Autodesk Inventor part; units mm, degrees
ref_plane "YZ Plane" through (0, 0, 0) normal (1, 0, 0) x (0, 1, 0)
ref_plane "XZ Plane" through (0, 0, 0) normal (0, 1, 0) x (-1, 0, 0)
ref_plane "XY Plane" through (0, 0, 0) normal (0, 0, 1) x (1, 0, 0)
sketch "Sketch1" plane through (0, 0, 0) normal (0, 1, 0) x (-1, 0, 0)
  line L0 (10.25, 29) -> (-10.25, 29)
  line L1 (-10.25, 29) -> (-10.25, -29)
  line L2 (-10.25, -29) -> (10.25, -29)
  line L3 (10.25, -29) -> (10.25, 29)
  line L4 (11.8375, 30.5875) -> (-11.8375, 30.5875)
  line L5 (-11.8375, 30.5875) -> (-11.8375, -30.5875)
  line L6 (-11.8375, -30.5875) -> (11.8375, -30.5875)
  line L7 (11.8375, -30.5875) -> (11.8375, 30.5875)
  point P0 (0, 0)
  dimension "d0" = 20.5
  dimension "d1" = 1.5875
  dimension "d2" = 1.5875
  dimension "d3" = 1.5875
  dimension "d4" = 1.5875
  dimension "d5" = 58
  dimension "d6" = 29
  dimension "d7" = 10.25
extrude "Extrusion1" add sketch "Sketch1" along normal blind 3.175
sketch "Sketch2" plane through (0, 0, 0) normal (0, -1, 0) x (1, 0, 0)
  line L0 (-10.25, -29) -> (-10.25, 29) construction
  line L1 (-10.25, 29) -> (10.25, 29) construction
  line L2 (10.25, 29) -> (10.25, -29) construction
  line L3 (10.25, -29) -> (-10.25, -29) construction
  line L4 (-11.8375, 30.5875) -> (11.8375, 30.5875)
  line L5 (-11.8375, -30.5875) -> (-11.8375, 30.5875)
  line L6 (11.8375, -30.5875) -> (-11.8375, -30.5875)
  line L7 (11.8375, 30.5875) -> (11.8375, -30.5875)
  point P0 (0, 0)
extrude "Extrusion2" add sketch "Sketch2" along normal blind 1.5875
sketch "Sketch3" plane through (0, 3.175, 0) normal (0, 1, 0) x (1, 0, 0)
  line L0 (11.8375, 30.5875) -> (11.8375, -30.5875)
  line L1 (10.25, -29) -> (10.25, 29)
  line L2 (-11.8375, -30.5875) -> (-11.8375, 30.5875)
  line L3 (-11.8375, -30.5875) -> (-10.2373, -30.5875)
  line L4 (-10.2373, -30.5875) -> (-10.2373, -5.1875)
  line L5 (-10.2373, -5.1875) -> (-11.8375, -5.1875)
  line L6 (-11.8375, -5.1875) -> (-11.8375, -30.5875)
  point P0 (0, 0)
  dimension "d13" = 1.6002
  dimension "d14" = 25.4
extrude "Extrusion3" add sketch "Sketch3" along normal blind 1.5875
equation "\"d2\" = d1"
equation "\"d3\" = d2"
equation "\"d4\" = d3"
properties part number "Camera Platform" material "Aluminum 6061"
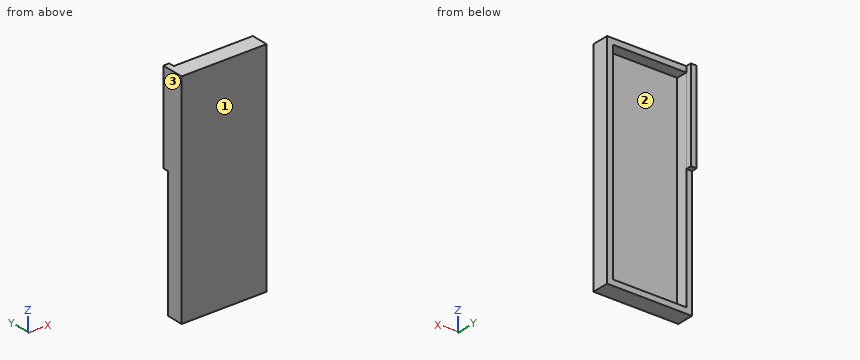
The listing builds one solid part. Answer for the finished solid, in the listing's coordinates (mm). Face numbers are marked on the shaded views. Give positions to 0.01 mm unless a question says otherwise; leave off trailing zeros. Loops run counter-clockwise (first coordinate to the right, second up) from the corner with the lowest first, then second, coordinate; pieces in that order, holes last. Notation, with made-up numbers: M 46.5,-38.75 L 67.5,-38.75 A16 ccw 67.5,-11.75 Z; hole C 57.25,86 d6. An arc over 180 degrees is marked long. One line per item, written item: value.
Q1. Determine the mould class of the marked faces 1, 2 and 3 for opening direction X: +X half, -X half, draft (parallel to the pull), parting line (faces both ways), or undercut.
Working result:
face 1: draft
face 2: undercut
face 3: -X half
Q2. A cutting plane is placed at C-C on x = 1.25. Determine the outline of the cut face in (y, z) (1 decimal).
Working result:
outline: M -1.6,-30.6 L 3.2,-30.6 L 3.2,-29 L 0,-29 L 0,29 L 3.2,29 L 3.2,30.6 L -1.6,30.6 Z
Q3. Find the intervals of material crossed by line 1 (Z direction, x = 2.75, y = 0.5); line 2 (X direction, y = 0.25, z = 0); line 3 (Y direction, x = 10.75, z = 5.5) (1 decimal), in increasing order. Write a range as from..to.
Working result:
line 1: z = -30.59..-29, 29..30.59
line 2: x = -11.84..-10.25, 10.25..11.84
line 3: y = -1.6..3.2
Q4. Flat-ended cylindrical pins translate along their axes: P1, Ø10, axis at x = -2.5, z = 0.5, coming from the +Y side; P2, Ø1.7, axis at x = -11, y = 4.5, coming from the -Z side. Find the tip coordinate at first contact, or state that the pin passes through.
Working result:
P1: stops at y = 0
P2: stops at z = 5.19
Q5. A cutting plane is placed at A-A on y = 1. Determine the outline of the cut face in (x, z), then the cut area to 3 significant figures.
Working result:
outline: M -11.84,-30.59 L 11.84,-30.59 L 11.84,30.59 L -11.84,30.59 Z; hole M -10.25,-29 L 10.25,-29 L 10.25,29 L -10.25,29 Z
area: 259 mm^2
